For this review, take the finished solid that the model builds, in its own axes (mm). Round coordinates to 2 decimals unless told otherwise and drop trailing zeros. Write each loop counter-clockwise with the first axis right and the second up, starting at its lowest first coordinate (ties: lowest second). Pieces come first, ordered by that corner, then holes. Notation, with made-up numbers: (25.5, 40) - (40.5, 40) arc R8 ccw to (40.5, 46) - close; hole circle Ø1 at (65, -16.5). An arc over 180 degrees is marked (long way). Answer in a Markdown table with one row per item. Add a question column.
from build123d import *

# Parameters (mm, degrees)
SKETCH1_R           = 6
SKETCH1_R_2         = 1.525
BOSS_EXTRUDE1_DEPTH = 5


with BuildPart() as part:
    # Sketch1 → Boss-Extrude1 (new body)
    with BuildSketch(Plane(origin=(0, 0, 0), x_dir=(1, 0, 0), z_dir=(0, 1, 0))):
        Polygon((0, -40.379460215), (80, -40.467284232), (80, -180), (0, -180), align=None)
        with Locations(Location((40, -131.25, 0), (0, 0, 270))):
            Circle(SKETCH1_R, mode=Mode.SUBTRACT)
        with Locations(Location((24.5, -138.25, 0), (0, 0, 270))):
            Circle(SKETCH1_R_2, mode=Mode.SUBTRACT)
        with Locations(Location((55.5, -138.25, 0), (0, 0, 270))):
            Circle(SKETCH1_R_2, mode=Mode.SUBTRACT)
        with Locations(Location((32.25, -124.826606241, 0), (0, 0, 270))):
            Circle(SKETCH1_R_2, mode=Mode.SUBTRACT)
        with Locations(Location((47.75, -124.826606241, 0), (0, 0, 270))):
            Circle(SKETCH1_R_2, mode=Mode.SUBTRACT)
    extrude(amount=BOSS_EXTRUDE1_DEPTH)


solid = part.part
Q1. Draft analysis for pull direction X (two halves, no side actions). For faces 1 (the face through (49.262, 2.465, 124.628)), 2 (the face through (0, 2, 111)), 3 (the face through (41, 2, 180)), 4 (the face through (80, 2, 109)), state which applies: released by +X, released by -X, zero draft, split by the parting line, or undercut.
Q2. Add section B-B on x = 55.5. State the section outline as (y, z) points (3 decimals), then the cut area to 3 significant figures.
Q3. To check wall thickness, follow probe 1 along X at (y, z) = (2.25, 138.25) (3 decimals); probe 2 along X at (y, z) = (0.7, 139); probe 3 along X at (y, z) = (1.7, 131.25). State the ranges of each line that lie inside material, in increasing order.
Q4. Add section A-A on x = 24.5. State the section outline as (y, z) points (3 decimals), then the cut area to 3 significant figures.
Q5. Insertion check: pin 1 Ø2.5 at (x, z) = (32.25, 124.83) entering from -Y; pin 2 Ø3 at (x, y) = (68, 3) entering from -Z. Each pin has a flat end and moves straight along its axis. Give the tip position at first contact, or say it passes through.
Answer sheet:
| question | item | result |
|---|---|---|
| 1 | face 1 | undercut |
| 1 | face 2 | released by -X |
| 1 | face 3 | zero draft |
| 1 | face 4 | released by +X |
| 2 | outline | (0, 40.44) - (5, 40.44) - (5, 136.725) - (0, 136.725) - close; (0, 139.775) - (5, 139.775) - (5, 180) - (0, 180) - close |
| 2 | area | 683 mm² |
| 3 | probe 1 | x = 0 to 22.975, 26.025 to 53.975, 57.025 to 80 |
| 3 | probe 2 | x = 0 to 23.17, 25.83 to 54.17, 56.83 to 80 |
| 3 | probe 3 | x = 0 to 34, 46 to 80 |
| 4 | outline | (0, 40.406) - (5, 40.406) - (5, 136.725) - (0, 136.725) - close; (0, 139.775) - (5, 139.775) - (5, 180) - (0, 180) - close |
| 4 | area | 683 mm² |
| 5 | pin 1 | passes through |
| 5 | pin 2 | stops at z = 40.45 |
